Answer from the drawing. Dimensions are ordinates in mm from the lowest x, y and z of the part. Coordinates: 2 decimals unless noted, no trailing zeros. Write each loop counter-clockwise with the first axis right and the second up, starting at its lowest first coordinate (ties: lowest second). Pieces come first, ordered by that corner, then holes.
(1) Section A-A on z = 75 is taken. Write down the section's boundary in (x, y), then the cut area to 3 significant figures.
(2) Find the intervals of material crossed by probe 1 along Z at (x, y) = (75, 0.9); probe 2 along Z at (x, y) = (31.5, 0.25), in increasing order.
(3) Given pin 1 (1 mm diameter, centred on y = 0.5, z = 125, fed in from -X); pin 2 (4.5 mm diameter, centred on x = 75, z = 75, fed in from -Y), each flat-ended and moving along its own axis, determine where each tip first touches the part or whether it passes through.
(4) Section C-C on x = 115.5 is taken. Write down the section's boundary in (y, z).
(5) Section B-B on x = 75 is taken. Write down the section's boundary in (y, z), then the cut area to 3 significant figures.
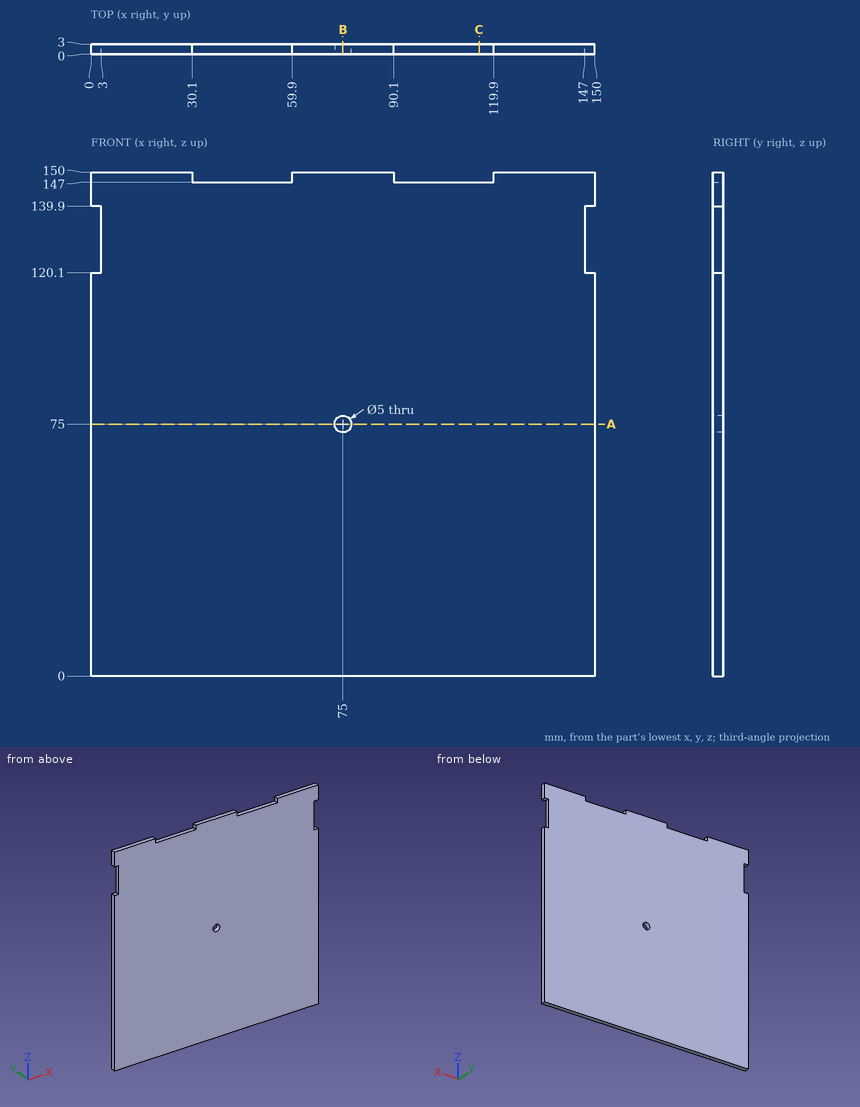
Response:
1. outline: (0, 0) - (72.5, 0) - (72.5, 3) - (0, 3) - close; (77.5, 0) - (150, 0) - (150, 3) - (77.5, 3) - close
1. area: 435 mm2
2. probe 1: z = 0 to 72.5, 77.5 to 150
2. probe 2: z = 0 to 147
3. pin 1: stops at x = 3
3. pin 2: passes through
4. outline: (0, 0) - (3, 0) - (3, 147) - (0, 147) - close
5. outline: (0, 0) - (3, 0) - (3, 72.5) - (0, 72.5) - close; (0, 77.5) - (3, 77.5) - (3, 150) - (0, 150) - close
5. area: 435 mm2
